Verification items for the finished model (mm, model axes). Face numbers are marked on the shaded views. A direction names the side the tool comes from. Coordinates: 2 decimals unless noted, no trailing zeros. Order: outer loops, then holes, each group sorted by start corner. A loop starts at its lowest first (then second) coordinate and runs counter-clockwise, first axis right, second up.
Q1. Cross-section at C-C, the plane z = 0.3. Record the boundary of the cut face in (x, y), and give its area (3 significant figures).
Q2. Thickness scan on line 1 (Y direction, x = -6, z = 2.4); line 2 (X direction, y = 4.75, z = 0.7); line 3 (Y direction, x = -6, z = 1.2). Record the ranges inside material, lowest first.
Q3. Draft check along Y on the marked faces 1, 2, 3 and 4. Enter one of: pulls with the +Y half, pulls with the -Y half, needs draft (parallel to the pull), parting line crosses it, or undercut.
Q4. Cross-section at D-D, the plane y = 8.75. Record the boundary of the cut face in (x, z), and give its area (3 significant figures).
Q5. Cross-section at B-B, the plane x = 6. Record the boundary of the cut face in (y, z), and give its area (3 significant figures).
Q6. Cross-section at A-A, the plane y = 5. Record the boundary of the cut face in (x, z), and give its area (3 significant figures).
Q7. Depth check by flat-ended pin: P1, Ø1.4, axis at x = -6, y = 5, coming from the +Z side; P2, Ø2, axis at x = 0, z = 2.5, coming from the +Y side; P3, Ø5, axis at x = 1, y = 7.5, coming from the -Z side; P4, Ø1.3, axis at x = 5.5, y = 4, coming from the +Z side. Enter the tip coordinate at first touch or a pass-through.
Q8. Set-up check for the marked faces 5, 6 and 7: record each of +Z, -Z, +X, -X, +Y, -Y from which the full face is reachable in a straight line by a thin tool's end or side.
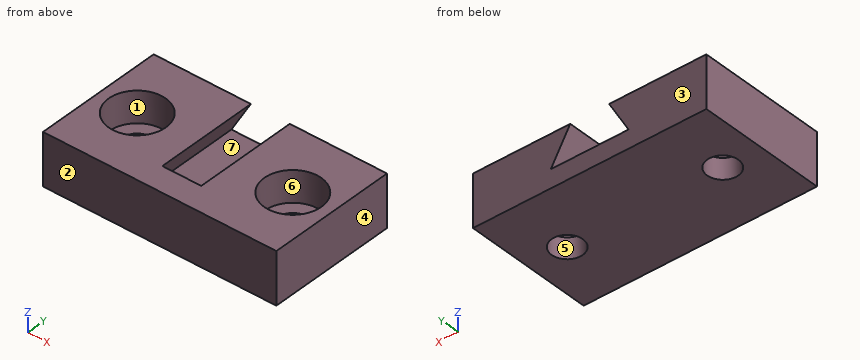
from build123d import *

# Parameters (mm, degrees)
BOSS_EXTRUDE1_DEPTH                                 = 10
BOSS_EXTRUDE2_DEPTH                                 = 2
CBORE_FOR_M2_HEX_SOCKET_HEAD_CAP_SCREW1_D           = 2.4
CBORE_FOR_M2_HEX_SOCKET_HEAD_CAP_SCREW1_CBORE_D     = 4.4
CBORE_FOR_M2_HEX_SOCKET_HEAD_CAP_SCREW1_CBORE_DEPTH = 2.4


with BuildPart() as part:
    # Sketch1 → Boss-Extrude1 (new body)
    with BuildSketch(Plane(origin=(0, 0, 0), x_dir=(1, 0, 0), z_dir=(0, 1, 0))):
        Polygon((-9, 0), (9, 0), (9, -4), (1.5, -4), (3, -1.401923789), (-3, -1.401923789), (-1.5, -4), (-9, -4), align=None)
    extrude(amount=BOSS_EXTRUDE1_DEPTH)

    # Sketch2 → Boss-Extrude2 (add)
    with BuildSketch(Plane.XZ):
        Polygon((-1.5, 4), (1.5, 4), (3, 1.401923789), (0.56541664, 1.071774791), (-3, 1.401923789), align=None)
    extrude(amount=-BOSS_EXTRUDE2_DEPTH)

    # CBORE for M2 Hex Socket Head Cap Screw1 (through all)
    with Locations(Plane.XY.offset(4)):
        with Locations((-6, 5), (6, 5)):
            CounterBoreHole(CBORE_FOR_M2_HEX_SOCKET_HEAD_CAP_SCREW1_D / 2, CBORE_FOR_M2_HEX_SOCKET_HEAD_CAP_SCREW1_CBORE_D / 2, CBORE_FOR_M2_HEX_SOCKET_HEAD_CAP_SCREW1_CBORE_DEPTH)


solid = part.part
Check values:
1. outline: (-9, 0) - (9, 0) - (9, 10) - (-9, 10) - close; hole circle Ø2.4 at (-6, 5); hole circle Ø2.4 at (6, 5)
1. area: 171 mm2
2. line 1: y = 0 to 2.8, 7.2 to 10
2. line 2: x = -9 to -7.17, -4.83 to 4.83, 7.17 to 9
2. line 3: y = 0 to 3.8, 6.2 to 10
3. face 1: undercut
3. face 2: pulls with the -Y half
3. face 3: pulls with the +Y half
3. face 4: needs draft
4. outline: (-9, 0) - (9, 0) - (9, 4) - (1.5, 4) - (3, 1.4) - (-3, 1.4) - (-1.5, 4) - (-9, 4) - close
4. area: 60.3 mm2
5. outline: (0, 0) - (3.8, 0) - (3.8, 1.6) - (2.8, 1.6) - (2.8, 4) - (0, 4) - close; (6.2, 0) - (10, 0) - (10, 4) - (7.2, 4) - (7.2, 1.6) - (6.2, 1.6) - close
5. area: 25.6 mm2
6. outline: (-9, 0) - (-7.2, 0) - (-7.2, 1.6) - (-8.2, 1.6) - (-8.2, 4) - (-9, 4) - close; (-4.8, 0) - (4.8, 0) - (4.8, 1.6) - (3.8, 1.6) - (3.8, 4) - (1.5, 4) - (3, 1.4) - (-3, 1.4) - (-1.5, 4) - (-3.8, 4) - (-3.8, 1.6) - (-4.8, 1.6) - close; (7.2, 0) - (9, 0) - (9, 4) - (8.2, 4) - (8.2, 1.6) - (7.2, 1.6) - close
6. area: 31.5 mm2
7. P1: passes through
7. P2: stops at y = 2
7. P3: stops at z = 0
7. P4: stops at z = 1.6
8. face 5: +Z, -Z
8. face 6: +Z
8. face 7: +Y
